```python
from build123d import *

# Parameters (mm, degrees)
F1_DEPTH       = 9
F2_DEPTH       = 9
F4_D           = 3.5
F4_CSINK_D     = 5
F4_CSINK_ANGLE = 90


with BuildPart() as f1:
    # F0 (on Right) → F1 (new body)
    with BuildSketch(Plane.YZ):
        with BuildLine():
            ThreePointArc((-5, -24.8), (-1.464466, -23.335534), (0, -19.8))
            Line((0, -19.8), (0, -14.8))
            ThreePointArc((0, -14.8), (-1.464466, -18.335534), (-5, -19.8))
            Line((-5, -19.8), (-24.8, -19.8))
            ThreePointArc((-24.8, -19.8), (-28.335534, -18.335534), (-29.8, -14.8))
            Line((-29.8, -14.8), (-29.8, -19.8))
            ThreePointArc((-29.8, -19.8), (-28.335534, -23.335534), (-24.8, -24.8))
            Line((-24.8, -24.8), (-5, -24.8))
        make_face()
        with BuildLine():
            ThreePointArc((-5, -19.8), (-1.464466, -18.335534), (0, -14.8))
            Line((0, -14.8), (0, 0))
            Line((0, 0), (-8.9, 0))
            Line((-8.9, 0), (-8.9, -5.8))
            ThreePointArc((-8.9, -5.8), (-14.9, -11.8), (-20.9, -5.8))
            Line((-20.9, -5.8), (-20.9, 0))
            Line((-20.9, 0), (-29.8, 0))
            Line((-29.8, 0), (-29.8, -14.8))
            ThreePointArc((-29.8, -14.8), (-28.335534, -18.335534), (-24.8, -19.8))
            Line((-24.8, -19.8), (-5, -19.8))
        make_face()
    extrude(amount=F1_DEPTH)

    # F0 (on Right) → F2 (join)
    with BuildSketch(Plane.YZ):
        with BuildLine():
            ThreePointArc((-5, -19.8), (-1.464466, -18.335534), (0, -14.8))
            Line((0, -14.8), (0, 0))
            Line((0, 0), (-8.9, 0))
            Line((-8.9, 0), (-8.9, -5.8))
            ThreePointArc((-8.9, -5.8), (-14.9, -11.8), (-20.9, -5.8))
            Line((-20.9, -5.8), (-20.9, 0))
            Line((-20.9, 0), (-29.8, 0))
            Line((-29.8, 0), (-29.8, -14.8))
            ThreePointArc((-29.8, -14.8), (-28.335534, -18.335534), (-24.8, -19.8))
            Line((-24.8, -19.8), (-5, -19.8))
        make_face()
    extrude(amount=-F2_DEPTH)

    # F4 (through all)
    with Locations(Plane.YZ.offset(9)):
        with Locations((-21.9, -22.3), (-7.9, -22.3)):
            CounterSinkHole(F4_D / 2, F4_CSINK_D / 2, counter_sink_angle=F4_CSINK_ANGLE)


solid = f1.part
```
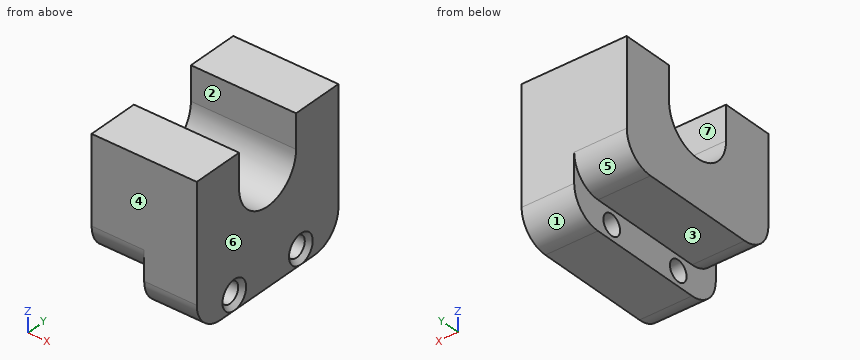
For this review, take the finished solid that the model builds, in its own axes (mm). Face numbers are marked on the shaded views. A direction names the side the tool comes from. Coordinates: 2 decimals unless noted, no trailing zeros. Write each loop counter-clockwise with the first axis right and the second up, starting at its lowest first coordinate (ties: lowest second). Pieces come first, ordered by that corner, then holes. Notation, with made-up numbers: (23, 67) - (66, 67) arc R15 cw to (66, 89) - close; hole circle Ø10 at (-38.5, 38.5). An arc over 180 degrees is marked (long way). Put each result on its own line as item: value.
1. Add section A-A, the plane z = -5. Give the boundary of the cut face in (x, y), then the cut area to 3 significant figures.
Values found:
outline: (-9, -29.8) - (9, -29.8) - (9, -20.9) - (-9, -20.9) - close; (-9, -8.9) - (9, -8.9) - (9, 0) - (-9, 0) - close
area: 320 mm²
2. For pin 1 (1.5 mm diameter, centred on x = -6, y = -16.5, fed in from +Z); pin 2 (4.5 mm diameter, centred on y = -7.9, z = -22.3, fed in from -X), all flat-tipped, find the tip position at first contact; note any pin that passes through.
Values found:
pin 1: z = -11.32
pin 2: x = 0
3. Mouldability with a two-part tool opening along Y and no side actions: class the marked faces 4, 5, 6 and 7 as released by +Y, released by -Y, zero draft, split by the parting line, or undercut.
Values found:
face 4: released by -Y
face 5: released by +Y
face 6: zero draft
face 7: undercut
4. Add section B-B, the plane x = 2. Give the boundary of the cut face in (y, z), then the cut area to 3 significant figures.
Values found:
outline: (-29.8, -19.8) arc R5 ccw to (-24.8, -24.8) - (-5, -24.8) arc R5 ccw to (0, -19.8) - (0, 0) - (-8.9, 0) - (-8.9, -5.8) arc R6 cw to (-20.9, -5.8) - (-20.9, 0) - (-29.8, 0) - close; hole circle Ø3.5 at (-21.9, -22.3); hole circle Ø3.5 at (-7.9, -22.3)
area: 583 mm²
5. Wall thickness on probe 1 along Y at (x, z) = (6.75, -22.3); probe 2 along Z at (x, y) = (2.5, -21.9); probe 3 along Y at (x, z) = (7.5, -1.25): over which ranges is each line inside the solid? List them lowest first.
Values found:
probe 1: -29.13 to -23.65, -20.15 to -9.65, -6.15 to -0.67
probe 2: -24.8 to -24.05, -20.55 to 0
probe 3: -29.8 to -20.9, -8.9 to 0
6. Add section D-D, the plane z = -22.3. Give the boundary of the cut face in (x, y).
Values found:
outline: (0, -29.13) - (9, -29.13) - (9, -24.4) - (8.25, -23.65) - (0, -23.65) - close; (0, -20.15) - (8.25, -20.15) - (9, -19.4) - (9, -10.4) - (8.25, -9.65) - (0, -9.65) - close; (0, -6.15) - (8.25, -6.15) - (9, -5.4) - (9, -0.67) - (0, -0.67) - close
7. Add section C-C, the plane x = -7. Give the boundary of the cut face in (y, z).
Values found:
outline: (-29.8, -14.8) arc R5 ccw to (-24.8, -19.8) - (-5, -19.8) arc R5 ccw to (0, -14.8) - (0, 0) - (-8.9, 0) - (-8.9, -5.8) arc R6 cw to (-20.9, -5.8) - (-20.9, 0) - (-29.8, 0) - close
8. Machinability: for the marked faces 1, 2 and 3, which of the approach directions +Z, -Z, +X, -X, +Y, -Y give a long, thin tool a straight path to every point of the face, cutting with its end or side? Answer none if there is none.
Values found:
face 1: -Z, +X, -X, +Y
face 2: +Z, +X, -X
face 3: -Z, -X, +Y, -Y
